Can you work these out from the model? Positions are in its coordinate system, mm. Give positions to 0.01 mm unless a question says otherwise; leave off trailing zeros. Order: outer loops, then holes, each group sorted by start corner. A loop starts at its lowest first (then second) coordinate and runs counter-clockwise, first axis right, second up.
Item 1: I want a section at B-B, the plane y = -44. Write out the boundary of the cut face in (x, z), then the cut area to 3 significant figures.
Item 2: If I drill on line 1 along X through (y, z) = (-27, -3); line 2 along Y through (x, z) = (273, -7); line 3 along X through (y, z) = (-80, -5), over which ranges is the centre line in solid material (lowest first)?
Item 3: I want a section at A-A, the plane x = 149. Write out the boundary of the cut face in (y, z).
Item 4: I'm going to push flat-ended pins straight in: pin 1 Ø4.5 at (x, y) = (208, 2) entering from -Z; pin 2 Ø1.2 at (x, y) = (93.5, 3) entering from -Z; pin 3 Ø1.5 at (x, y) = (40.5, -25.5) entering from -Z. Where does each tip first touch, or does it pass through?
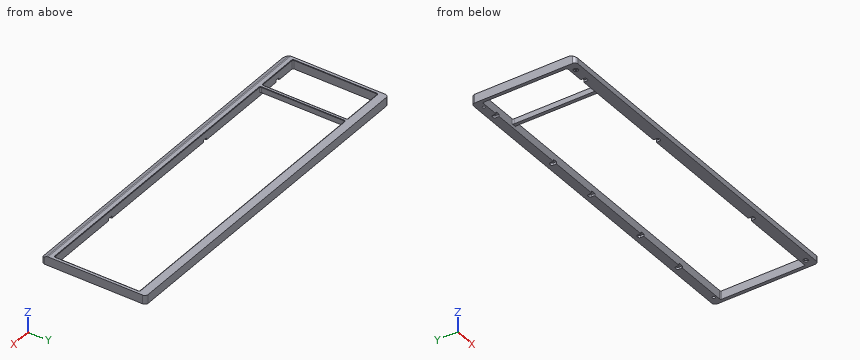
```python
from build123d import *

# Parameters (mm, degrees)
SKETCH3_W                      = 316.5625
SKETCH3_H                      = 95.2
BOSS_EXTRUDE1_DEPTH            = 8
SKETCH3_3_W                    = 3
SKETCH3_3_H                    = 67.175
SKETCH3_3_H_2                  = 10.025
BOSS_EXTRUDE2_DEPTH            = 5
CHAMFER1_SIZE                  = 3
CHAMFER1_SIZE2                 = 5.196152423
FILLET3_R                      = 3
CUT_EXTRUDE1_DEPTH             = 2
FILLET1_R                      = 3
FILLET5_R                      = 1
CHAMFER2_SIZE                  = 0.5
CHAMFER2_SIZE2                 = 0.288675135
FILLET6_R                      = 0.5
CBORE_FOR_M2_SHCS2_D           = 2.4
CBORE_FOR_M2_SHCS2_DEPTH       = 12.278967257
CBORE_FOR_M2_SHCS2_CBORE_D     = 4.4
CBORE_FOR_M2_SHCS2_CBORE_DEPTH = 4
CBORE_FOR_M2_SHCS2_TIP         = 0.721032743
CBORE_FOR_M2_SHCS3_D           = 2.4
CBORE_FOR_M2_SHCS3_DEPTH       = 8.278967257
CBORE_FOR_M2_SHCS3_CBORE_D     = 4.4
CBORE_FOR_M2_SHCS3_CBORE_DEPTH = 3
CBORE_FOR_M2_SHCS3_TIP         = 0.721032743


with BuildPart() as part:
    # Sketch3 → Boss-Extrude1 (new body)
    with BuildSketch(Plane.XY):
        with Locations((154.78125, -39.1)):
            Rectangle(SKETCH3_W, SKETCH3_H)
        Polygon((38.98125, -76.7), (41.98125, -76.7), (310.0625, -76.7), (310.0625, 0.5), (41.98125, 0.5), (38.98125, 0.5), (-0.5, 0.5), (-0.5, -76.7), align=None, mode=Mode.SUBTRACT)
    extrude(amount=-BOSS_EXTRUDE1_DEPTH)

    # Sketch3<3> → Boss-Extrude2 (add)
    with BuildSketch(Plane.XY):
        with Locations((40.48125, -43.1125)):
            Rectangle(SKETCH3_3_W, SKETCH3_3_H)
        with Locations((40.48125, -4.5125)):
            Rectangle(SKETCH3_3_W, SKETCH3_3_H_2)
    extrude(amount=-BOSS_EXTRUDE2_DEPTH)

    # Chamfer1
    chamfer1_edges = [part.edges().sort_by_distance(p)[0] for p in [
        (154.78125, -86.7, 0),
    ]]
    chamfer1_side = [part.faces().sort_by_distance(p)[0] for p in [
        (154.78125, -86.7, -4),
    ]]
    chamfer(chamfer1_edges, length=CHAMFER1_SIZE, length2=CHAMFER1_SIZE2, reference=chamfer1_side[0])

    # Fillet3
    fillet3_edges = [part.edges().sort_by_distance(p)[0] for p in [
        (154.78125, -81.503847577, 0),
    ]]
    fillet(fillet3_edges, radius=FILLET3_R)

    # Sketch8 → Cut-Extrude1 (cut)
    with BuildSketch(Plane(origin=(0, 0, -8), x_dir=(-1, 0, 0), z_dir=(0, 0, -1))):
        with BuildLine():
            Line((-260.0625, 0.5), (-260.0625, 3.5))
            ThreePointArc((-260.0625, 3.5), (-259.623160172, 4.560660172), (-258.5625, 5))
            Line((-258.5625, 5), (-257.5625, 5))
            ThreePointArc((-257.5625, 5), (-256.501839828, 4.560660172), (-256.0625, 3.5))
            Line((-256.0625, 3.5), (-256.0625, 0.5))
            Line((-256.0625, 0.5), (-260.0625, 0.5))
        make_face()
        with BuildLine():
            Line((-115.98125, -76.7), (-115.98125, -79.7))
            ThreePointArc((-115.98125, -79.7), (-115.541910172, -80.760660172), (-114.48125, -81.2))
            Line((-114.48125, -81.2), (-113.48125, -81.2))
            ThreePointArc((-113.48125, -81.2), (-112.420589828, -80.760660172), (-111.98125, -79.7))
            Line((-111.98125, -79.7), (-111.98125, -76.7))
            Line((-111.98125, -76.7), (-115.98125, -76.7))
        make_face()
        with BuildLine():
            Line((-210.0625, 0.5), (-210.0625, 3.5))
            ThreePointArc((-210.0625, 3.5), (-209.623160172, 4.560660172), (-208.5625, 5))
            Line((-208.5625, 5), (-207.5625, 5))
            ThreePointArc((-207.5625, 5), (-206.501839828, 4.560660172), (-206.0625, 3.5))
            Line((-206.0625, 3.5), (-206.0625, 0.5))
            Line((-206.0625, 0.5), (-210.0625, 0.5))
        make_face()
        with BuildLine():
            Line((-145.98125, 0.5), (-145.98125, 3.5))
            ThreePointArc((-145.98125, 3.5), (-145.541910172, 4.560660172), (-144.48125, 5))
            Line((-144.48125, 5), (-143.48125, 5))
            ThreePointArc((-143.48125, 5), (-142.420589828, 4.560660172), (-141.98125, 3.5))
            Line((-141.98125, 3.5), (-141.98125, 0.5))
            Line((-141.98125, 0.5), (-145.98125, 0.5))
        make_face()
        with BuildLine():
            Line((-95.98125, 0.5), (-95.98125, 3.5))
            ThreePointArc((-95.98125, 3.5), (-95.541910172, 4.560660172), (-94.48125, 5))
            Line((-94.48125, 5), (-93.48125, 5))
            ThreePointArc((-93.48125, 5), (-92.420589828, 4.560660172), (-91.98125, 3.5))
            Line((-91.98125, 3.5), (-91.98125, 0.5))
            Line((-91.98125, 0.5), (-95.98125, 0.5))
        make_face()
        with BuildLine():
            Line((-21.240625, 0.5), (-21.240625, 3.5))
            ThreePointArc((-21.240625, 3.5), (-20.801285172, 4.560660172), (-19.740625, 5))
            Line((-19.740625, 5), (-18.740625, 5))
            ThreePointArc((-18.740625, 5), (-17.679964828, 4.560660172), (-17.240625, 3.5))
            Line((-17.240625, 3.5), (-17.240625, 0.5))
            Line((-17.240625, 0.5), (-21.240625, 0.5))
        make_face()
        with BuildLine():
            Line((-239.5625, -76.7), (-239.5625, -79.7))
            ThreePointArc((-239.5625, -79.7), (-239.123160172, -80.760660172), (-238.0625, -81.2))
            Line((-238.0625, -81.2), (-237.0625, -81.2))
            ThreePointArc((-237.0625, -81.2), (-236.001839828, -80.760660172), (-235.5625, -79.7))
            Line((-235.5625, -79.7), (-235.5625, -76.7))
            Line((-235.5625, -76.7), (-239.5625, -76.7))
        make_face()
        with BuildLine():
            Line((-21.240625, -76.7), (-21.240625, -79.7))
            ThreePointArc((-21.240625, -79.7), (-20.801285172, -80.760660172), (-19.740625, -81.2))
            Line((-19.740625, -81.2), (-18.740625, -81.2))
            ThreePointArc((-18.740625, -81.2), (-17.679964828, -80.760660172), (-17.240625, -79.7))
            Line((-17.240625, -79.7), (-17.240625, -76.7))
            Line((-17.240625, -76.7), (-21.240625, -76.7))
        make_face()
    extrude(amount=-CUT_EXTRUDE1_DEPTH, mode=Mode.SUBTRACT)

    # Fillet1
    fillet1_edges = [part.edges().sort_by_distance(p)[0] for p in [
        (313.0625, -86.7, -5.5),
        (-3.5, -86.7, -5.5),
        (-3.5, 8.5, -4),
        (313.0625, 8.5, -4),
    ]]
    fillet(fillet1_edges, radius=FILLET1_R)

    # Fillet5
    fillet5_edges = [part.edges().sort_by_distance(p)[0] for p in [
        (310.0625, -76.7, -4),
        (310.0625, 0.5, -4),
        (-0.5, 0.5, -4),
        (-0.5, -76.7, -4),
        (41.98125, 0.5, -2.5),
        (41.98125, -76.7, -2.5),
        (38.98125, -76.7, -2.5),
        (38.98125, 0.5, -2.5),
    ]]
    fillet(fillet5_edges, radius=FILLET5_R)

    # Chamfer2
    chamfer2_edges = [part.edges().sort_by_distance(p)[0] for p in [
        (310.0625, -38.1, 0),
        (19.240625, -76.7, 0),
        (176.021875, -76.7, 0),
        (176.021875, 0.5, 0),
        (19.240625, 0.5, 0),
        (41.98125, -38.1, 0),
        (38.98125, -38.1, 0),
        (-0.5, -38.1, 0),
        (309.769606781, -76.407106781, 0),
        (309.769606781, 0.207106781, 0),
        (42.274143219, 0.207106781, 0),
        (42.274143219, -76.407106781, 0),
        (38.688356781, -76.407106781, 0),
        (-0.207106781, -76.407106781, 0),
        (-0.207106781, 0.207106781, 0),
        (38.688356781, 0.207106781, 0),
    ]]
    chamfer2_side = [part.faces().sort_by_distance(p)[0] for p in [
        (310.391389733, -38.1, 0),
    ]]
    chamfer(chamfer2_edges, length=CHAMFER2_SIZE, length2=CHAMFER2_SIZE2, reference=chamfer2_side[0])

    # Fillet6
    fillet6_edges = [part.edges().sort_by_distance(p)[0] for p in [
        (256.0625, 0.5, -7),
        (260.0625, 0.5, -7),
    ]]
    fillet(fillet6_edges, radius=FILLET6_R)

    # CBORE for M2 SHCS2
    with Locations(Plane(origin=(0, -0.720708302, -17.082674747), x_dir=(-1, 0, 0), z_dir=(0, 0, -1))):
        with Locations((-304.78125, 3.743540113), (-4.78125, 3.743540113)):
            CounterBoreHole(CBORE_FOR_M2_SHCS2_D / 2, CBORE_FOR_M2_SHCS2_CBORE_D / 2, CBORE_FOR_M2_SHCS2_CBORE_DEPTH, depth=CBORE_FOR_M2_SHCS2_DEPTH)
            with Locations((0, 0, -(CBORE_FOR_M2_SHCS2_DEPTH + CBORE_FOR_M2_SHCS2_TIP / 2))):  # 118° drill point
                Cone(0, CBORE_FOR_M2_SHCS2_D / 2, CBORE_FOR_M2_SHCS2_TIP, mode=Mode.SUBTRACT)

    # CBORE for M2 SHCS3
    with Locations(Plane(origin=(0, 0, -9.799622892), x_dir=(1, 0, 0), z_dir=(0, 0, -1))):
        with Locations((4.78125, 80.87420884), (304.78125, 80.87420884)):
            CounterBoreHole(CBORE_FOR_M2_SHCS3_D / 2, CBORE_FOR_M2_SHCS3_CBORE_D / 2, CBORE_FOR_M2_SHCS3_CBORE_DEPTH, depth=CBORE_FOR_M2_SHCS3_DEPTH)
            with Locations((0, 0, -(CBORE_FOR_M2_SHCS3_DEPTH + CBORE_FOR_M2_SHCS3_TIP / 2))):  # 118° drill point
                Cone(0, CBORE_FOR_M2_SHCS3_D / 2, CBORE_FOR_M2_SHCS3_TIP, mode=Mode.SUBTRACT)


solid = part.part
```
Results list:
1. outline: (-3.5, -8) - (-0.5, -8) - (-0.5, -0.29) - (-1, 0) - (-3.5, 0) - close; (38.98, -5) - (41.98, -5) - (41.98, -0.29) - (41.48, 0) - (39.48, 0) - (38.98, -0.29) - close; (310.06, -8) - (313.06, -8) - (313.06, 0) - (310.56, 0) - (310.06, -0.29) - close
1. area: 62.7 mm2
2. line 1: x = -3.5 to -0.5, 38.98 to 41.98, 310.06 to 313.06
2. line 2: y = -86.7 to -76.7, 0.5 to 8.5
2. line 3: x = -3.5 to 3.96, 5.6 to 303.96, 305.6 to 313.06
3. outline: (-86.7, -8) - (-76.7, -8) - (-76.7, -0.29) - (-77.2, 0) - (-80.7, 0) arc R3 ccw to (-82.2, -0.4) - (-86.7, -3) - close; (0.5, -8) - (8.5, -8) - (8.5, 0) - (1, 0) - (0.5, -0.29) - close
4. pin 1: stops at z = -8
4. pin 2: stops at z = -6
4. pin 3: stops at z = -5
